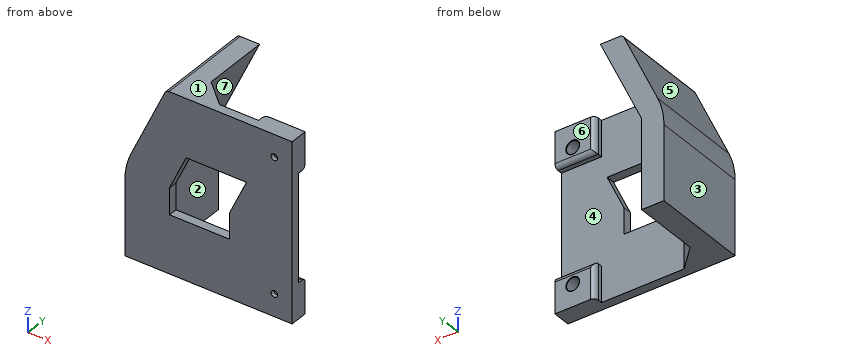
```python
from build123d import *

# Parameters (mm, degrees)
SKETCH_1_W               = 57
SKETCH_1_H               = 80
EXTRUDE_1_DEPTH          = 4
EXTRUDE_2_DEPTH          = 40
CUT_EXTRUDE_1_DEPTH      = 16
SKETCH_4_W               = 80
SKETCH_4_H               = 4
EXTRUDE_3_DEPTH          = 20
SKETCH_7_W               = 20
SKETCH_7_H               = 80
EXTRUDE_4_DEPTH          = 4
CUT_EXTRUDE_2_DEPTH      = 4
CUT_EXTRUDE_2_DEPTH_BACK = 4
SKETCH_5_R               = 1.45
SKETCH_8_R               = 2.9
CUT_EXTRUDE_3_DEPTH      = 6
SKETCH_9_W               = 80
SKETCH_9_H               = 8
CUT_EXTRUDE_4_DEPTH      = 2
SKETCH_10_W              = 18
SKETCH_10_H              = 48
CUT_EXTRUDE_5_DEPTH      = 4
CUT_EXTRUDE_6_DEPTH      = 4
CHAMFER_1_SIZE           = 10
FILLET_1_R               = 30
FILLET_2_R               = 2
FILLET_3_R               = 0.2


with BuildPart() as part:
    # 草图1 → 凸台-拉伸1 (new body)
    with BuildSketch(Plane(origin=(0, 0, 0), x_dir=(1, 0, 0), z_dir=(0, 1, 0))):
        with Locations((-28.5, 40)):
            Rectangle(SKETCH_1_W, SKETCH_1_H)
    extrude(amount=EXTRUDE_1_DEPTH)

    # 草图2 → 凸台-拉伸2 (add)
    with BuildSketch(Plane(origin=(0, 4, 0), x_dir=(1, 0, 0), z_dir=(0, 1, 0))):
        Polygon((-47, 40), (-28.5, 0), (-38.5, 0), (-57, 40), (-57, 80), (-47, 80), align=None)
    extrude(amount=EXTRUDE_2_DEPTH)

    # 草图3 → 切除-拉伸1 (cut)
    with BuildSketch(Plane(origin=(0, 4, 0), x_dir=(1, 0, 0), z_dir=(0, 1, 0))):
        Polygon((-38.5, 0), (-57, 40), (-57, 0), align=None)
    extrude(amount=-CUT_EXTRUDE_1_DEPTH, mode=Mode.SUBTRACT)

    # 草图4 → 凸台-拉伸3 (add)
    with BuildSketch(Plane(origin=(0, 0, 0), x_dir=(0, 0, -1), z_dir=(1, 0, 0))):
        with Locations((40, 2)):
            Rectangle(SKETCH_4_W, SKETCH_4_H)
    extrude(amount=EXTRUDE_3_DEPTH)

    # 草图7 → 凸台-拉伸4 (add)
    with BuildSketch(Plane(origin=(0, 4, 0), x_dir=(1, 0, 0), z_dir=(0, 1, 0))):
        with Locations((10, 40)):
            Rectangle(SKETCH_7_W, SKETCH_7_H)
    extrude(amount=EXTRUDE_4_DEPTH)

    # 草图5 → 切除-拉伸2 (cut, two sides: drawn at the far end of the back side and taken through both)
    with BuildSketch(Plane(origin=(0, 4, 0), x_dir=(1, 0, 0), z_dir=(0, 1, 0)).offset(-CUT_EXTRUDE_2_DEPTH_BACK)):
        with Locations(Location((10, 70, 0), (0, 0, 270))):
            Circle(SKETCH_5_R)
        with Locations(Location((10, 10, 0), (0, 0, 90))):
            Circle(SKETCH_5_R)
    extrude(amount=CUT_EXTRUDE_2_DEPTH + CUT_EXTRUDE_2_DEPTH_BACK, mode=Mode.SUBTRACT)

    # 草图8 → 切除-拉伸3 (cut)
    with BuildSketch(Plane(origin=(0, 8, 0), x_dir=(1, 0, 0), z_dir=(0, 1, 0))):
        with Locations(Location((10, 70, 0), (0, 0, 270))):
            Circle(SKETCH_8_R)
        with Locations(Location((10, 10, 0), (0, 0, 270))):
            Circle(SKETCH_8_R)
    extrude(amount=-CUT_EXTRUDE_3_DEPTH, mode=Mode.SUBTRACT)

    # 草图9 → 切除-拉伸4 (cut)
    with BuildSketch(Plane(origin=(20, 0, 0), x_dir=(0, 0, -1), z_dir=(1, 0, 0))):
        with Locations((40, 4)):
            Rectangle(SKETCH_9_W, SKETCH_9_H)
    extrude(amount=-CUT_EXTRUDE_4_DEPTH, mode=Mode.SUBTRACT)

    # 草图10 → 切除-拉伸5 (cut)
    with BuildSketch(Plane(origin=(0, 8, 0), x_dir=(1, 0, 0), z_dir=(0, 1, 0))):
        with Locations((9, 40)):
            Rectangle(SKETCH_10_W, SKETCH_10_H)
    extrude(amount=-CUT_EXTRUDE_5_DEPTH, mode=Mode.SUBTRACT)

    # 草图11 → 切除-拉伸6 (cut)
    with BuildSketch(Plane(origin=(0, 4, 0), x_dir=(1, 0, 0), z_dir=(0, 1, 0))):
        Polygon((-37, 42.200521891), (-29.507258625, 26), (-2.507258625, 26), (-10, 42.200521891), (-10, 54), (-37, 54), align=None)
    extrude(amount=-CUT_EXTRUDE_6_DEPTH, mode=Mode.SUBTRACT)

    # 倒角1
    chamfer_1_edges = [part.edges().sort_by_distance(p)[0] for p in [
        (-37.75, 4, -20),
        (-47, 4, -60),
    ]]
    chamfer(chamfer_1_edges, length=CHAMFER_1_SIZE - 0.0001)  # a hair under: the kernel refuses the full size

    # 圆角1
    fillet_1_edges = [part.edges().sort_by_distance(p)[0] for p in [
        (-57, 22, -40),
    ]]
    fillet(fillet_1_edges, radius=FILLET_1_R)

    # 圆角2
    fillet_2_edges = [part.edges().sort_by_distance(p)[0] for p in [
        (0, 8, -8),
        (9, 8, -16),
        (9, 8, -64),
        (-38.5, 22, 0),
        (0, 8, -72),
    ]]
    fillet(fillet_2_edges, radius=FILLET_2_R)

    # 圆角3
    fillet_3_edges = [part.edges().sort_by_distance(p)[0] for p in [
        (10, 2, -71.45),
        (10, 8, -72.9),
        (10, 2, -8.55),
        (10, 8, -12.9),
    ]]
    fillet(fillet_3_edges, radius=FILLET_3_R)


solid = part.part
```
The model under review builds one solid part; all positions refer to its coordinate system, in mm. Face numbers are marked on the shaded views. A direction names the side the tool comes from. Give positions to 0.01 mm unless a question says otherwise; leave off trailing zeros. Write each loop counter-clockwise with the first axis right and the second up, starting at its lowest first coordinate (ties: lowest second). Pieces come first, ordered by that corner, then holes. Notation, with made-up numbers: (-29.75, 16) - (-13.75, 16) arc R19 cw to (-13.75, 51) - close; hole circle Ø5 at (8, 64.25). An arc over 180 degrees is marked (long way). Answer in a Markdown table with one row per item. Add a question column.
1. We need section D-D on z = -55. Write out the cut boundary in (x, y), then the cut area to 3 significant figures.
2. We need section C-C on x = 10. State how many separate pieces and enclosed holes the cut face has, then the cut area to 3 significant figures.
3. Draft analysis for pull direction X (two halves, no side actions). For the marked faces 1, 2, 3 and 4, state which applies: +X half, -X half, draft (parallel to the pull), parting line (faces both ways), or undercut.
4. We need section B-B on y = 24.5. Write out the cut boundary in (x, z).
5. Tool access review of the marked faces 5, 6 and 7: name each direction out of +Z, -Z, +X, -X, +Y, -Y from which nothing blocks a thin tool from reaching the whole face with its end or side.
6. Wall thickness on line 1 along Z through (x, y) = (10, 1.1); line 2 along X through (y, z) = (6, -70); line 3 along Y through (x, z) = (-3, -24): over which ranges is each line inside the solid? List them lowest first. Write a range as [from, to].
7. We need section A-A on z = -70. Write out the cut boundary in (x, y), then the cut area to 3 significant figures.
8. Insertion check: P1, Ø4, axis at x = 2, z = -58, coming from the +Y side; P2, Ø2, axis at x = -37, y = 26, coming from the -Z side; P3, Ø8, axis at y = 15, z = -65.5, coming from the +X side. Each pin has a flat end and moves straight along its axis. Give the tip position at first contact, or say it passes through.
Ans:
| question | item | result |
|---|---|---|
| 1 | outline | (-57, 0) - (18, 0) - (18, 4) - (-37, 4) - (-47, 14) - (-47, 44) - (-57, 44) - close |
| 1 | area | 750 mm^2 |
| 2 | separate pieces | 3 |
| 2 | enclosed holes | 0 |
| 2 | area | 365 mm^2 |
| 3 | face 1 | draft |
| 3 | face 2 | +X half |
| 3 | face 3 | -X half |
| 3 | face 4 | undercut |
| 4 | outline | (-57, -80) - (-47, -80) - (-47, -40) - (-28.5, 0) - (-37.22, 0) arc R2 ccw to (-39.04, -1.16) - (-54.23, -34.01) arc R30 ccw to (-57, -46.6) - close |
| 5 | face 5 | +Z, -X, +Y, -Y |
| 5 | face 6 | +Z, -Z, +X, +Y |
| 5 | face 7 | -Z, +X, +Y |
| 6 | line 1 | z = [-80, -71.45], [-68.55, -11.45], [-8.55, 0] |
| 6 | line 2 | x = [-57, -39], [0, 7.1], [12.9, 18] |
| 6 | line 3 | y = [0, 4] |
| 7 | outline | (-57, 0) - (8.55, 0) - (8.55, 1.8) arc R0.2 ccw to (8.35, 2) - (7.1, 2) - (7.1, 7.8) arc R0.2 ccw to (6.9, 8) - (2, 8) arc R2 ccw to (0, 6) - (0, 4) - (-37, 4) - (-47, 14) - (-47, 44) - (-57, 44) - close; (11.45, 0) - (18, 0) - (18, 8) - (13.1, 8) arc R0.2 ccw to (12.9, 7.8) - (12.9, 2) - (11.65, 2) arc R0.2 ccw to (11.45, 1.8) - close |
| 7 | area | 781 mm^2 |
| 8 | P1 | stops at y = 4 |
| 8 | P2 | stops at z = -20.54 |
| 8 | P3 | stops at x = -44 |
